Input: part model. Units: mm. Frame: model coordinates. A direction names the side the tool comes from. Coordinates: 2 decimals unless noted, no trailing zeros. Order: outer loops, then holes, each group sorted by start corner. A loop starts at its lowest first (then second) coordinate and runs counter-clockwise, first axis right, second up. Notation, with made-up numbers: (83.5, 79) - (90.5, 79) arc R13 ccw to (90.5, 86) - close; hole circle Ø1 at (-24, -23.5). An arc over 180 degrees is marked (long way). Use a Markdown table: item, result. Add a question column.
from build123d import *

# Parameters (mm, degrees)
SKETCH_1_R          = 22
EXTRUDE_1_DEPTH     = 22
SKETCH_2_R          = 10
CUT_EXTRUDE_1_DEPTH = 5
CHAMFER_1_SIZE      = 1
SKETCH_3_R          = 0.911044844
CUT_EXTRUDE_2_DEPTH = 1
CHAMFER_2_SIZE      = 0.9


with BuildPart() as part:
    # 草图1 → 凸台-拉伸1 (new body)
    with BuildSketch(Plane.XY):
        Circle(SKETCH_1_R)
    extrude(amount=EXTRUDE_1_DEPTH)

    # 草图2 → 切除-拉伸1 (cut)
    with BuildSketch(Plane.XY.offset(22)):
        Circle(SKETCH_2_R)
    extrude(amount=-CUT_EXTRUDE_1_DEPTH, mode=Mode.SUBTRACT)

    # 倒角1
    chamfer_1_edges = [part.edges().sort_by_distance(p)[0] for p in [
        (-22, 0, 0),
        (-22, 0, 22),
    ]]
    chamfer(chamfer_1_edges, length=CHAMFER_1_SIZE)

    # 草图3 → 切除-拉伸2 (cut)
    with BuildSketch(Plane(origin=(0, 0, 0), x_dir=(-1, 0, 0), z_dir=(0, 0, -1))):
        with Locations((0, 18.818302181)):
            Circle(SKETCH_3_R)
    extrude(amount=-CUT_EXTRUDE_2_DEPTH, mode=Mode.SUBTRACT)

    # 倒角2
    chamfer_2_edges = [part.edges().sort_by_distance(p)[0] for p in [
        (0.911044844, 18.818302181, 1),
    ]]
    chamfer(chamfer_2_edges, length=CHAMFER_2_SIZE)


solid = part.part
1) Cut plane C-C (z = 15.75). Return the cut outline in (x, y), and give its area (3 significant figures).
2) Reachability of faces 1 (the conical face through (0.03, 19.07, 0.76)), 2 (the flat face through (0, 0, 17)) from +Z, -Z, +X, -X, +Y, -Y: full face, straight path, thin tool, end or side. Return the list, or none.
3) Cut plane A-A (z = 20). Return the cut outline in (x, y), and give its area (3 significant figures).
4) Contact query for flat-ended pins moving along their axis: P1, Ø5, axis at y = 10, z = 17.5, coming from the +X side; P2, Ø3, axis at y = 8, z = 10, coming from the -X side; P3, Ø12, axis at x = 7.5, z = 12.5, coming from the +Y side. Output: stop coordinate, or through.
5) Cut plane B-B (y = 0). Return the cut outline in (x, z).
6) Material intervals for L1, parallel to Y at x = 0, z = 18.85; L2, parallel to Z at x = 1, y = -8; L3, parallel to Y at x = 0, z = 0.05, sorted ascending.
7) Pull-direction query (X, two-part tool) for faces 3 (the cylindrical face through (-4.769, -21.477, 10.86)), 4 (the flat face through (9, 5, 22)), 5 (the cylindrical face through (-2.17, -9.76, 19.54)); classes: pulls with the +X half, pulls with the -X half, needs draft (parallel to the pull), parting line crosses it, or undercut.
Computed:
| question | item | result |
|---|---|---|
| 1 | outline | circle Ø44 at (0, 0) |
| 1 | area | 1,520 mm2 |
| 2 | face 1 | -Z |
| 2 | face 2 | +Z |
| 3 | outline | circle Ø44 at (0, 0); hole circle Ø20 at (0, 0) |
| 3 | area | 1,210 mm2 |
| 4 | P1 | stops at x = 20.68 |
| 4 | P2 | stops at x = -21.02 |
| 4 | P3 | stops at y = 21.95 |
| 5 | outline | (-22, 1) - (-21, 0) - (21, 0) - (22, 1) - (22, 21) - (21, 22) - (10, 22) - (10, 17) - (-10, 17) - (-10, 22) - (-21, 22) - (-22, 21) - close |
| 6 | L1 | y = -22 to -10, 10 to 22 |
| 6 | L2 | z = 0 to 17 |
| 6 | L3 | y = -21.05 to 17.91, 19.73 to 21.05 |
| 7 | face 3 | parting line crosses it |
| 7 | face 4 | needs draft |
| 7 | face 5 | undercut |
